from build123d import *

# Parameters (mm, degrees)
PAD_DEPTH     = 1
SKETCH001_R   = 9.7
SKETCH001_R_2 = 9.1
PAD001_DEPTH  = 3


with BuildPart() as part:
    # Sketch → Pad (new body)
    with BuildSketch(Plane.XY):
        Polygon((10, 0.1), (10, -9.9), (0, -9.9), (0, -6.5), (3.4, -6.5), (3.4, -8.1), (6.5, -8.1), (6.5, -1.8), (3.4, -1.8), (3.4, -3.4), (0, -3.4), (0, 0), (0, 59.4), (39.6, 59.4), (39.6, 0), (39.6, -3.6), (43.2, -3.6), (43.2, -2.2), (46, -2.2), (46, -7.7), (43.2, -7.7), (43.2, -6.3), (39.6, -6.3), (39.6, -9.9), (37, -9.9), (37, 0.1), align=None)
    extrude(amount=-PAD_DEPTH)

    # Sketch001 → Pad001 (join)
    with BuildSketch(Plane.XY):
        with Locations((9.9, 9.9)):
            Circle(SKETCH001_R)
        with Locations((9.9, 9.9)):
            Circle(SKETCH001_R_2, mode=Mode.SUBTRACT)
    extrude(amount=PAD001_DEPTH)


solid = part.part
Here's how the part is built. I have some questions about the finished solid (model axes, mm). A direction names the side the tool comes from. Round coordinates to 2 decimals unless told otherwise and drop trailing zeros. Order: outer loops, then holes, each group sorted by start corner. A loop starts at its lowest first (then second) coordinate and runs counter-clockwise, first axis right, second up. Notation, with made-up numbers: M 54.5,81 L 89.5,81 A22 cw 89.5,106 Z; hole C 28.5,49 d6. An arc over 180 degrees is marked long. Return JSON: item names as keys, results as strings. Group by question number.
1. If we section it at B-B on y = 9.9: List the corners of the cut face in (x, z) for me, then the cut area to 3 significant figures.
2. Please list where these lines run through material, in increasing order: probe 1 along Y at (x, z) = (10, 0.8); probe 2 along Z at (x, y) = (35, 47); probe 3 along X at (y, z) = (41.5, -0.6).
3. If we section it at A-A on z = 2.05: List the corners of the cut face in (x, y) for me.
4. If we section it at C-C on x = 41.5: List the corners of the cut face in (y, z) for me.
5. If we mould it in two halves opening along X, with no side actions, what happens to faces 3 (the face through (14.099, 1.827, 1.479)), 4 (the face through (2.2, 4, 1.5)), 5 (the face through (1, 7, 3))? For each: pulls with the +X half, pulls with the -X half, needs draft (parallel to the pull), parting line crosses it, or undercut.
6. I'm going to push flat-ended pins straight in: pin 1 Ø0.8 at (x, z) = (42, -0.5) entering from +Y; pin 2 Ø0.5 at (x, z) = (28.5, -0.5) entering from -Y; pin 3 Ø1.1 at (x, z) = (41.5, -0.5) entering from -Y. Where does each tip first touch, or does it pass through?
7. If we section it at D-D on y = 41.5: List the corners of the cut face in (x, z) for me, then the cut area to 3 significant figures.
8. On a 3-axis mill with a long thin cutter (end or side, diameter ignored), from which of +Z, -Z, +X, -X, +Y, -Y can I reach the whole of each face in a straight line? I mean faces 1 (the face through (10, 10, 0)), 2 (the face through (23, 25, -1)). Say none if no direction works.
Reply:
{
 "1": {"outline": "M 0,-1 L 39.6,-1 L 39.6,0 L 19.6,0 L 19.6,3 L 19,3 L 19,0 L 0.8,0 L 0.8,3 L 0.2,3 L 0.2,0 L 0,0 Z", "area": "43.2 mm^2"},
 "2": {"probe 1": "0.2 to 0.8, 19 to 19.6", "probe 2": "-1 to 0", "probe 3": "0 to 39.6"},
 "3": {"outline": "C 9.9,9.9 d19.4; hole C 9.9,9.9 d18.2"},
 "4": {"outline": "M -6.3,-1 L -3.6,-1 L -3.6,0 L -6.3,0 Z"},
 "5": {"face 3": "undercut", "face 4": "parting line crosses it", "face 5": "needs draft"},
 "6": {"pin 1": "y = -3.6", "pin 2": "y = 0.1", "pin 3": "y = -6.3"},
 "7": {"outline": "M 0,-1 L 39.6,-1 L 39.6,0 L 0,0 Z", "area": "39.6 mm^2"},
 "8": {"face 1": "+Z", "face 2": "-Z, +X, -X, +Y, -Y"}
}
